```python
from build123d import *

# Parameters (mm, degrees)
SCHNITT_LINEAR_AUSTRAGEN1_DEPTH = 27.567610021


with BuildPart() as part:
    # Austragung1: sweep along a path in SK Pfad
    with BuildLine(Plane(origin=(0, 0, 0), x_dir=(0, 0, -1), z_dir=(0.843391446, -0.537299608, 0))) as austragung1_path:
        Line((0, 0), (50.603486749, 32.237976501))
    # SK Grundriss → Austragung1 (sweep)
    with BuildSketch(Plane.XY):
        Polygon((0, 0), (54.378467222, 25.357095704), (54.378467222, 85.357095704), (0, 60), align=None)
    sweep(path=austragung1_path.line)

    # Skizze2 → Schnitt-Linear austragen1 (cut, through all)
    with BuildSketch(Plane(origin=(58.655853729, 92.071247611, -39.620266542), x_dir=(0.863081214, -0.463933603, 0.199640751), z_dir=(0.505065162, 0.7927935, -0.341156339))):
        Polygon((15.113369899, 15.241721945), (-20.07640222, 7.593557233), (3.904191248, -17.963473004), align=None)
    extrude(amount=SCHNITT_LINEAR_AUSTRAGEN1_DEPTH, mode=Mode.SUBTRACT)


solid = part.part
```
Could you check a few things on this model? Use its own coordinates, in mm. Give positions to 0.01 mm unless a question says otherwise; leave off trailing zeros. Order: outer loops, then holes, each group sorted by start corner. A loop starts at its lowest first (then second) coordinate and runs counter-clockwise, first axis right, second up.
Q1. If I drill on line 1 along X through (y, z) = (50, -35); line 2 along Y through (x, z) = (50.5, -23.5); line 3 along X through (y, z) = (80, -32), over which ranges is the centre line in solid material (lowest first)?
Q2. Suppose I cut it at B-B, the plane x = 43.5. Write out the boundary of the cut face in (y, z).
Q3. Suppose I cut it at A-A, the plane y = 73. Write out the boundary of the cut face in (x, z).
Q4. Suppose I cut it at D-D, the plane y = 84. Write out the boundary of the cut face in (x, z).
Q5. Suppose I cut it at C-C, the plane z = -8. Write out the boundary of the cut face in (x, y).
Q6. I'm going to push flat-ended pins straight in: P1, Ø1.5, axis at x = 60.5, z = -40, coming from the +Y side; P2, Ø4, axis at y = 68, z = -16.5, coming from the -X side; P3, Ø4, axis at y = 29.5, z = -22.5, coming from the -X side. Where does each tip first touch, or does it pass through?
Solution:
1. line 1: x = 11.98 to 66.36
1. line 2: y = 32.42 to 92.42
1. line 3: x = 16.97 to 65.33
2. outline: (20.28, 0) - (39.4, -50.6) - (97, -50.6) - (98.28, -47.64) - (80.28, 0) - close
3. outline: (8.28, -24.2) - (17.32, -50.6) - (71.7, -50.6) - (54.38, 0) - (27.88, 0) - close
4. outline: (15.29, -44.67) - (17.32, -50.6) - (63.91, -50.6) - (69.08, -42.95) - (54.38, 0) - (51.47, 0) - close
5. outline: (2.74, 4.3) - (57.12, 29.66) - (57.12, 89.66) - (2.74, 64.3) - close
6. P1: stops at y = 91.31
6. P2: stops at x = 4.97
6. P3: stops at x = 7.02
